The listing builds one solid part. Answer for the finished solid, in the listing's coordinates (mm). A direction names the side the tool comes from. Coordinates: 2 decimals unless noted, no trailing zeros. Order: outer loops, then holes, each group sorted by start corner. A loop starts at its lowest first (then second) coordinate and runs counter-clockwise, first axis right, second up. Notation, with made-up numbers: (80, 46) -> (87, 46) arc R8 ccw to (87, 57) -> close; hole circle Ø8 at (-11, -15.75). An arc over 180 degrees is marked (long way). Write item = value, one per line.
from build123d import *

# Parameters (mm, degrees)
SKETCH1_W           = 161
SKETCH1_H           = 145
BOSS_EXTRUDE1_DEPTH = 3
BOSS_EXTRUDE2_DEPTH = 15
CUT_EXTRUDE1_DEPTH  = 3
CUT_EXTRUDE2_DEPTH  = 2
CUT_EXTRUDE3_DEPTH  = 12
CUT_EXTRUDE5_DEPTH  = 12
CUT_EXTRUDE6_DEPTH  = 20
CUT_EXTRUDE8_DEPTH  = 10
FILLET2_R           = 5
FILLET3_R           = 5
SKETCH11_R          = 1.5
SKETCH11_R_2        = 1.25
CUT_EXTRUDE9_DEPTH  = 10


with BuildPart() as part:
    # Sketch1 → Boss-Extrude1 (new body)
    with BuildSketch(Plane(origin=(0, 0, 0), x_dir=(1, 0, 0), z_dir=(0, 1, 0))):
        with Locations((-80.5, 0)):
            Rectangle(SKETCH1_W, SKETCH1_H)
    extrude(amount=BOSS_EXTRUDE1_DEPTH)

    # Sketch2 → Boss-Extrude2 (add)
    with BuildSketch(Plane(origin=(0, 0, 0), x_dir=(1, 0, 0), z_dir=(0, 1, 0))):
        Polygon((0, 72.5), (0, 84.5), (-173, 84.5), (-173, -84.5), (0, -84.5), (0, -72.5), (-161, -72.5), (-161, 72.5), align=None)
    extrude(amount=BOSS_EXTRUDE2_DEPTH)

    # Sketch3 → Cut-Extrude1 (cut)
    with BuildSketch(Plane(origin=(0, 15, 0), x_dir=(1, 0, 0), z_dir=(0, 1, 0))):
        Polygon((-161, 44.1), (-161, 37.8), (-164.3, 37.8), (-164.3, 12.95), (-168.8, 12.95), (-168.8, 68.95), (-164.3, 68.95), (-164.3, 44.1), align=None)
        Polygon((-24.95, -75.8), (-49.8, -75.8), (-49.8, -72.5), (-56.1, -72.5), (-56.1, -75.8), (-80.95, -75.8), (-80.95, -80.3), (-24.95, -80.3), align=None)
        Polygon((-161, -38.5), (-161, -44.8), (-164.3, -44.8), (-164.3, -65.1), (-168.8, -65.1), (-168.8, -18.2), (-164.3, -18.2), (-164.3, -38.5), align=None)
        Polygon((-99.75, -80.3), (-99.75, -75.8), (-124.6, -75.8), (-124.6, -72.5), (-130.9, -72.5), (-130.9, -75.8), (-155.75, -75.8), (-155.75, -80.3), align=None)
        Polygon((-48.3, 75.8), (-48.3, 72.5), (-54.6, 72.5), (-54.6, 75.8), (-79.45, 75.8), (-79.45, 80.3), (-23.45, 80.3), (-23.45, 75.8), align=None)
    extrude(amount=-CUT_EXTRUDE1_DEPTH, mode=Mode.SUBTRACT)

    # Sketch4 → Cut-Extrude2 (cut)
    with BuildSketch(Plane(origin=(0, 12, 0), x_dir=(1, 0, 0), z_dir=(0, 1, 0))):
        Polygon((-54.6, 72.5), (-48.3, 72.5), (-48.3, 75.8), (-42.0875, 75.8), (-42.0875, 80.3), (-60.8125, 80.3), (-60.8125, 75.8), (-54.6, 75.8), align=None)
        Polygon((-161, 44.1), (-161, 37.8), (-164.3, 37.8), (-164.3, 27.850226284), (-168.8, 27.850226284), (-168.8, 50.3125), (-164.3, 50.3125), (-164.3, 44.1), align=None)
        Polygon((-168.8, -33.425), (-168.8, -49.875), (-164.3, -49.875), (-164.3, -44.8), (-161, -44.8), (-161, -38.5), (-164.3, -38.5), (-164.3, -33.425), align=None)
        Polygon((-130.9, -72.5), (-130.9, -75.8), (-137.1125, -75.8), (-137.1125, -80.3), (-118.3875, -80.3), (-118.3875, -75.8), (-124.6, -75.8), (-124.6, -72.5), align=None)
        Polygon((-56.1, -75.8), (-62.3125, -75.8), (-62.3125, -80.3), (-43.5875, -80.3), (-43.5875, -75.8), (-49.8, -75.8), (-49.8, -72.5), (-56.1, -72.5), align=None)
    extrude(amount=-CUT_EXTRUDE2_DEPTH, mode=Mode.SUBTRACT)

    # Sketch5 → Cut-Extrude3 (cut)
    with BuildSketch(Plane.ZY.offset(173)):
        with BuildLine():
            Line((-5.75, 10.5), (10.63, 10.5))
            ThreePointArc((10.63, 10.5), (13.63, 7.5), (10.63, 4.5))
            Line((10.63, 4.5), (-5.75, 4.5))
            ThreePointArc((-5.75, 4.5), (-8.75, 7.5), (-5.75, 10.5))
        make_face()
    extrude(amount=-CUT_EXTRUDE3_DEPTH, mode=Mode.SUBTRACT)

    # Sketch7 → Cut-Extrude5 (cut)
    with BuildSketch(Plane(origin=(0, 0, -84.5), x_dir=(-1, 0, 0), z_dir=(0, 0, -1))):
        with BuildLine():
            Line((-4.5375, 10.634328206), (11.8425, 10.634328206))
            ThreePointArc((11.8425, 10.634328206), (14.8425, 7.634328206), (11.8425, 4.634328206))
            Line((11.8425, 4.634328206), (-4.5375, 4.634328206))
            ThreePointArc((-4.5375, 4.634328206), (-7.5375, 7.634328206), (-4.5375, 10.634328206))
        make_face()
    extrude(amount=-CUT_EXTRUDE5_DEPTH, mode=Mode.SUBTRACT)

    # Sketch8 → Cut-Extrude6 (cut)
    with BuildSketch(Plane(origin=(0, 0, -84.5), x_dir=(-1, 0, 0), z_dir=(0, 0, -1))):
        with BuildLine():
            Line((137.86, 11.4), (146.86, 11.4))
            ThreePointArc((146.86, 11.4), (151.36, 6.9), (146.86, 2.4))
            Line((146.86, 2.4), (137.86, 2.4))
            ThreePointArc((137.86, 2.4), (133.36, 6.9), (137.86, 11.4))
        make_face()
    extrude(amount=-CUT_EXTRUDE6_DEPTH, mode=Mode.SUBTRACT)

    # Sketch10 → Cut-Extrude8 (cut)
    with BuildSketch(Plane(origin=(0, 0, 0), x_dir=(0, 0, -1), z_dir=(1, 0, 0))):
        Polygon((-80.5, 15), (-76.5, 15), (-76.5, 11), (-72.5, 11), (-72.5, 7), (-76.5, 7), (-76.5, 3), (-80.5, 3), (-80.5, 7), (-84.5, 7), (-84.5, 11), (-80.5, 11), align=None)
    extrude(amount=-CUT_EXTRUDE8_DEPTH, mode=Mode.SUBTRACT)

    # Fillet2
    fillet2_edges = [part.edges().sort_by_distance(p)[0] for p in [
        (-173, 7.5, 84.5),
    ]]
    fillet(fillet2_edges, radius=FILLET2_R)

    # Fillet3
    fillet3_edges = [part.edges().sort_by_distance(p)[0] for p in [
        (-173, 7.5, -84.5),
    ]]
    fillet(fillet3_edges, radius=FILLET3_R)

    # Sketch11 → Cut-Extrude9 (cut)
    with BuildSketch(Plane(origin=(0, 0, 0), x_dir=(0, 0, -1), z_dir=(1, 0, 0))):
        with Locations((78.5, 2.317164103)):
            Circle(SKETCH11_R)
        with Locations((78.5, 12.817164103)):
            Circle(SKETCH11_R_2)
    extrude(amount=-CUT_EXTRUDE9_DEPTH, mode=Mode.SUBTRACT)


solid = part.part
Q1. Find the intervals of material crossed by line 1 along Y through (x, z) = (-7, -78.5); line 2 along Z through (x, y) = (-21.5, 3.5); line 3 along X through (y, z) = (12, -35.5), in increasing order.
The answers:
line_1 = 0 to 0.82, 3.82 to 4.63, 10.63 to 11.57, 14.07 to 15
line_2 = -84.5 to -72.5, 72.5 to 84.5
line_3 = -173 to -168.8, -164.3 to -161
Q2. The mould has two halves that part along Z. Classify faces 1 (the face through (-53, 13, 80.3)), 2 (the face through (-85, 7, 84.5)), 3 (the face through (-14.84, 7.7, -78.58)): released by +Z, released by -Z, zero draft, split by the parting line, or undercut.
The answers:
face_1 = undercut
face_2 = released by +Z
face_3 = zero draft
Q3. Each of these flat-tipped pins is pushed along its axis until it touches: pin 1 Ø3.5 at (y, z) = (2.5, -79) entering from +X; pin 2 Ø2 at (x, z) = (-167.5, 56.5) entering from +Y; pin 3 Ø4 at (y, z) = (13, -36.5) entering from +X; pin 4 Ø2 at (y, z) = (11.5, 78) entering from +X. Where does it stop, or does it pass through?
The answers:
pin_1 = 0
pin_2 = 12
pin_3 = -161
pin_4 = -10
Q4. A tool of negligible diameter and unlimited length cuts with its end or side. For faces 4 (the face through (-167, 12, -60)), 5 (the face through (-5, 5, 76.5)), 6 (the face through (-6, 4.634, -79)), from which of +Z, -Z, +X, -X, +Y, -Y can it reach the whole face along a straight path? Write none if from no direction.
The answers:
face_4 = +Y
face_5 = +X, +Y
face_6 = -Z, +X
Q5. Section A-A, the plane z = -57 is taken. Give the vertices of the cut face in (x, y), plus the area to 4 significant figures.
The answers:
outline = (-173, 0) -> (0, 0) -> (0, 3) -> (-161, 3) -> (-161, 15) -> (-164.3, 15) -> (-164.3, 12) -> (-168.8, 12) -> (-168.8, 15) -> (-173, 15) -> close
area = 649.5 mm2
